The listing builds one solid part. Answer for the finished solid, in the listing's coordinates (mm). Round coordinates to 2 decimals unless told otherwise and drop trailing zeros. Write each loop counter-clockwise with the first axis right and the second up, starting at its lowest first coordinate (ties: lowest second). Pieces come first, ordered by that corner, then holes.
(1) This flat-tipped pin is pushed along its axis until it touches: pin 1 Ø23 at (x, y) = (-79.59, 28.18) entering from +Z. Where does it stop, or does it pass through?
(2) A cutting plane is placed at C-C, the plane z = 0.65. Give the number of separate pieces and of enclosed holes in the cut face, and give its area (3 significant figures).
(3) Find the intervals of material crossed by probe 1 along X at (y, z) = (-17, 0.5); probe 2 along X at (y, z) = (29.5, 0.85); probe 3 along Y at (x, z) = (51.5, 0.5), in increasing order.
(4) A cutting plane is placed at A-A, the plane y = -10. Give the vertices of the cut face in (x, z).
(5) A cutting plane is placed at B-B, the plane x = 71.5. Give the vertices of the cut face in (y, z), and give its area (3 significant figures).
(6) A cutting plane is placed at D-D, the plane y = 15.5. Give the vertices of the cut face in (x, z).
from build123d import *

# Parameters (mm, degrees)
F0_R     = 19
F0_R_2   = 2.5
F1_DEPTH = 0.9
F3_DEPTH = 0.9


# Not quite as in the source:
# - the program builds the solid bodies; features that only make, move or delete a surface that nothing else refers to are left out


with BuildPart() as f1:
    # F0 (on Top) → F1 (new body)
    with BuildSketch(Plane.XY):
        Polygon((127.4130453914, 50.6848765003), (-102.5869546086, 50.6848765003), (-102.5869546086, 5.6848765003), (-102.5869546086, -39.3151234997), (-102.5869546086, -84.3151234997), (-56.5869546086, -84.3151234997), (-10.5869546086, -84.3151234997), (35.4130453914, -84.3151234997), (81.4130453914, -84.3151234997), (127.4130453914, -84.3151234997), align=None)
        with Locations((-79.5869546086, -61.8151234997)):
            Circle(F0_R, mode=Mode.SUBTRACT)
        with Locations((-33.5869546086, -61.8151234997)):
            Circle(F0_R, mode=Mode.SUBTRACT)
        with Locations((12.4130453914, -61.8151234997)):
            Circle(F0_R, mode=Mode.SUBTRACT)
        with Locations((-56.5869546086, -39.3151234997)):
            Circle(F0_R_2, mode=Mode.SUBTRACT)
        with Locations((-10.5869546086, -39.3151234997)):
            Circle(F0_R_2, mode=Mode.SUBTRACT)
        with Locations((58.7792091643, -61.8151234997)):
            Circle(F0_R, mode=Mode.SUBTRACT)
        with Locations((104.7792091643, -61.8151234997)):
            Circle(F0_R, mode=Mode.SUBTRACT)
        with Locations((35.4130453914, -39.3151234997)):
            Circle(F0_R_2, mode=Mode.SUBTRACT)
        with Locations((81.4130453914, -39.3151234997)):
            Circle(F0_R_2, mode=Mode.SUBTRACT)
        with Locations((-79.5869546086, -16.8151234997)):
            Circle(F0_R, mode=Mode.SUBTRACT)
        with Locations((-56.5869546086, 5.6848765003)):
            Circle(F0_R_2, mode=Mode.SUBTRACT)
        with Locations((-33.5869546086, -16.8151234997)):
            Circle(F0_R, mode=Mode.SUBTRACT)
        with Locations((12.4130453914, -15.8099713178)):
            Circle(F0_R, mode=Mode.SUBTRACT)
        with Locations((-10.5869546086, 5.6848765003)):
            Circle(F0_R_2, mode=Mode.SUBTRACT)
        with Locations((-79.5869546086, 28.1848765003)):
            Circle(F0_R, mode=Mode.SUBTRACT)
        with Locations((-33.5869546086, 28.1848765003)):
            Circle(F0_R, mode=Mode.SUBTRACT)
        with Locations((12.4130453914, 28.1848765003)):
            Circle(F0_R, mode=Mode.SUBTRACT)
        with Locations((58.7792091643, -15.8099713178)):
            Circle(F0_R, mode=Mode.SUBTRACT)
        with Locations((35.4130453914, 5.6848765003)):
            Circle(F0_R_2, mode=Mode.SUBTRACT)
        with Locations((104.7792091643, -16.8151234997)):
            Circle(F0_R, mode=Mode.SUBTRACT)
        with Locations((81.4130453914, 5.6848765003)):
            Circle(F0_R_2, mode=Mode.SUBTRACT)
        with Locations((59.1453729371, 28.1848765003)):
            Circle(F0_R, mode=Mode.SUBTRACT)
        with Locations((105.1453729371, 28.1848765003)):
            Circle(F0_R, mode=Mode.SUBTRACT)
    extrude(amount=F1_DEPTH)

    # F0 (on Top) → F3 (join)
    with BuildSketch(Plane.XY):
        with Locations((35.4130453914, -39.3151234997)):
            Circle(F0_R_2)
        with Locations((81.4130453914, -39.3151234997)):
            Circle(F0_R_2)
        with Locations((81.4130453914, 5.6848765003)):
            Circle(F0_R_2)
        with Locations((35.4130453914, 5.6848765003)):
            Circle(F0_R_2)
        with Locations((-10.5869546086, 5.6848765003)):
            Circle(F0_R_2)
        with Locations((-56.5869546086, 5.6848765003)):
            Circle(F0_R_2)
        with Locations((-56.5869546086, -39.3151234997)):
            Circle(F0_R_2)
        with Locations((-10.5869546086, -39.3151234997)):
            Circle(F0_R_2)
    extrude(amount=F3_DEPTH)


solid = f1.part
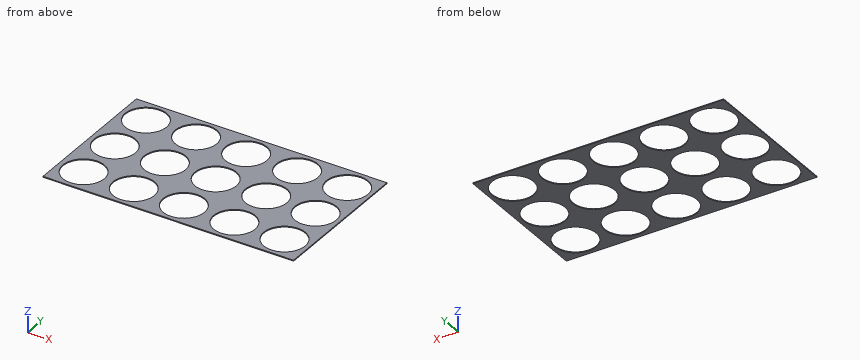
Solutions:
1. pin 1: passes through
2. separate pieces: 1
2. enclosed holes: 15
2. area: 14,000 mm2
3. probe 1: x = -102.59 to -98.59, -60.59 to -52.59, -14.59 to -6.55, 31.38 to 39.82, 77.74 to 85.78, 123.78 to 127.41
3. probe 2: x = -102.59 to -98.54, -60.63 to -52.54, -14.63 to -6.54, 31.37 to 40.19, 78.1 to 86.19, 124.1 to 127.41
3. probe 3: y = -84.32 to -79.37, -44.26 to -33.36, 1.74 to 10.79, 45.58 to 50.68
4. outline: (-102.59, 0) - (-97.32, 0) - (-97.32, 0.9) - (-102.59, 0.9) - close; (-61.85, 0) - (-51.32, 0) - (-51.32, 0.9) - (-61.85, 0.9) - close; (-15.85, 0) - (-5.68, 0) - (-5.68, 0.9) - (-15.85, 0.9) - close; (30.5, 0) - (40.69, 0) - (40.69, 0.9) - (30.5, 0.9) - close; (76.87, 0) - (87.04, 0) - (87.04, 0.9) - (76.87, 0.9) - close; (122.51, 0) - (127.41, 0) - (127.41, 0.9) - (122.51, 0.9) - close
5. outline: (-84.32, 0) - (-75.93, 0) - (-75.93, 0.9) - (-84.32, 0.9) - close; (-47.7, 0) - (-29.92, 0) - (-29.92, 0.9) - (-47.7, 0.9) - close; (-1.7, 0) - (13.75, 0) - (13.75, 0.9) - (-1.7, 0.9) - close; (42.62, 0) - (50.68, 0) - (50.68, 0.9) - (42.62, 0.9) - close
5. area: 44.7 mm2
6. outline: (-102.59, 0) - (-93.73, 0) - (-93.73, 0.9) - (-102.59, 0.9) - close; (-65.44, 0) - (-47.73, 0) - (-47.73, 0.9) - (-65.44, 0.9) - close; (-19.44, 0) - (-1.73, 0) - (-1.73, 0.9) - (-19.44, 0.9) - close; (26.56, 0) - (45, 0) - (45, 0.9) - (26.56, 0.9) - close; (73.29, 0) - (91, 0) - (91, 0.9) - (73.29, 0.9) - close; (119.29, 0) - (127.41, 0) - (127.41, 0.9) - (119.29, 0.9) - close
